Input: dimensioned drawing with shaded views. Units: mm. Origin: part minimum x, y, z. Give positions to 0.01 mm unless a question says otherwise; leave off trailing zeros. Write each loop counter-clockwise with the first axis right and the second up, starting at its lowest first coordinate (ties: lowest second). Pieces come first, ordered by that corner, then holes.
Q1. Mould query, pull axis Z, two halves, no side actions, for the marked faces 1, 2 and 3. Classes: +Z half, -Z half, draft (parallel to the pull), parting line (faces both ways), or undercut.
Q2. Section A-A (x = 8.5). Return the cut outline in (y, z).
Q3. Pin query (flat end, axial travel): pin 1 Ø2 at (y, z) = (2, 2) entering from +X; pin 2 Ø4 at (x, z) = (6.5, 5.5) entering from +Y; pin 3 Ø2 at (y, z) = (4.5, 4) entering from +X. Return the tip coordinate at first contact, or that it passes through.
Q4. Line query: line 1 (X direction, y = 5, z = 5.5); line 2 (X direction, y = 2, z = 0.75); line 3 (Y direction, x = 1.25, z = 1.5) (1 decimal). Output: solid intervals per line, ascending.
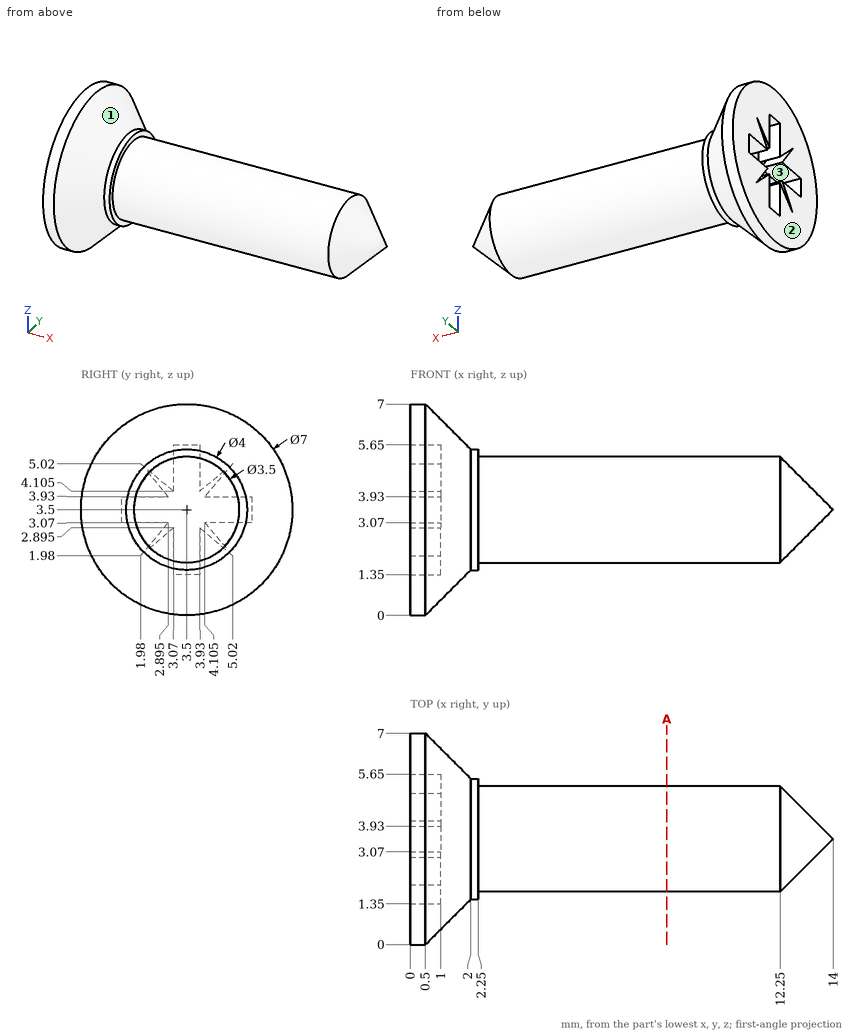
Computed:
1. face 1: parting line
1. face 2: draft
1. face 3: undercut
2. outline: circle Ø3.5 at (3.5, 3.5)
3. pin 1: stops at x = 12.88
3. pin 2: stops at y = 5.25
3. pin 3: stops at x = 13.88
4. line 1: x = 0 to 1.5
4. line 2: x = 0 to 0.87
4. line 3: y = 1.6 to 5.4
